Autodesk Inventor part; units mm, degrees
ref_plane "YZ Plane" through (0, 0, 0) normal (1, 0, 0) x (0, 1, 0)
ref_plane "XZ Plane" through (0, 0, 0) normal (0, 1, 0) x (-1, 0, 0)
ref_plane "XY Plane" through (0, 0, 0) normal (0, 0, 1) x (1, 0, 0)
sketch "Sketch1" plane through (0, 0, 0) normal (0, 0, 1) x (1, 0, 0)
  circle A0 centre (0, 0) radius 3.175
  circle A1 centre (0, 0) radius 12.7
  line L0 (-495.3, 0) -> (-495.3, 25.4)
  line L1 (-495.3, 25.4) -> (12.7, 25.4)
  line L2 (12.7, 25.4) -> (12.7, 0)
  line L3 (-12.7, 0) -> (-495.3, 0)
  dimension "d0" = 6.35
  dimension "d1" = 25.4
  dimension "d2" = 508
  dimension "d3" = 25.4
extrude "Extrusion1" add sketch "Sketch1" along normal blind 12.7
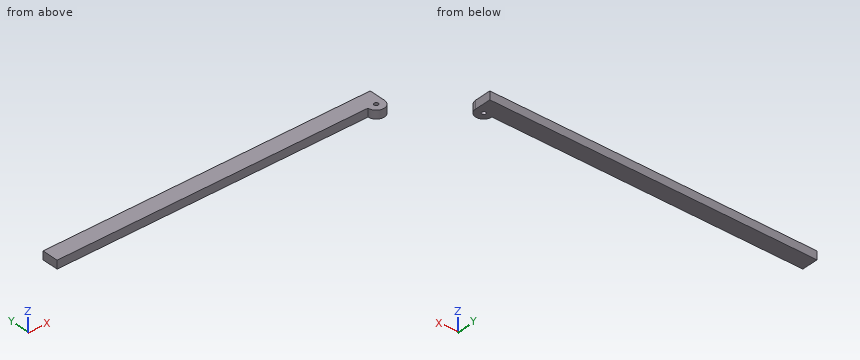
Geometry: final body of the model. Coordinates: model frame, mm. Give positions to 0.01 mm unless a question says otherwise; leave off trailing zeros. Write each loop counter-clockwise with the first axis right and the second up, starting at its lowest first coordinate (ties: lowest second). Pieces come first, ordered by that corner, then holes. Notation, with made-up numbers: (-38, -27.5) - (-10, -27.5) arc R24 cw to (-10, -15.5) - close; hole circle Ø5 at (-6.5, 61). An arc over 180 degrees is marked (long way). Return JSON: item names as keys, results as strings. Group by question number.
1) First-contact query: P1, Ø6.5, axis at x = -211.5, z = 4, coming from the -Y side; P2, Ø2, axis at y = -8, z = 5.5, coming from the -X side. Flat tips, straight axial feed; report the tip coordinate or a pass-through.
2) Line query: line 1 (Y direction, x = 0, z = 9.5) (3 decimals); line 2 (Y direction, x = -363, z = 6.75); line 3 (X direction, y = -6, z = 0.75). Output: solid intervals per line, ascending.
3) Section A-A on z = 6. Return the cut outline in (x, y) (3 decimals), plus the area to 3 significant figures.
4) Section B-B on x = -359. Return the cut outline in (y, z), plus the area to 3 significant figures.
Filled in:
{
 "1": {"P1": "stops at y = 0", "P2": "stops at x = -10.6"},
 "2": {"line 1": "y = -12.7 to -3.175, 3.175 to 25.4", "line 2": "y = 0 to 25.4", "line 3": "x = -11.19 to 11.19"},
 "3": {"outline": "(-495.3, 0) - (-12.7, 0) arc R12.7 ccw to (12.7, 0) - (12.7, 25.4) - (-495.3, 25.4) - close; hole circle Ø6.35 at (0, 0)", "area": "13,100 mm^2"},
 "4": {"outline": "(0, 0) - (25.4, 0) - (25.4, 12.7) - (0, 12.7) - close", "area": "323 mm^2"}
}
